```python
from build123d import *

# Parameters (mm, degrees)
SKETCH_1_W          = 8
SKETCH_1_H          = 5
EXTRUDE_1_DEPTH     = 5
SKETCH_2_W          = 1
SKETCH_2_H          = 2
EXTRUDE_2_DEPTH     = 5
EXTRUDE_3_DEPTH     = 1
SKETCH_7_W          = 8
SKETCH_7_H          = 1.5
EXTRUDE_4_DEPTH     = 1
CUT_EXTRUDE_2_DEPTH = 11.677078252
CUT_EXTRUDE_3_DEPTH = 10
CUT_EXTRUDE_4_DEPTH = 10
SKETCH_11_R         = 1.25
CUT_EXTRUDE_5_DEPTH = 1


with BuildPart() as part:
    # 草图1 → 凸台-拉伸1 (new body)
    with BuildSketch(Plane.XY):
        with Locations((0, 2.5)):
            Rectangle(SKETCH_1_W, SKETCH_1_H)
    extrude(amount=EXTRUDE_1_DEPTH)

    # 草图2 → 凸台-拉伸2 (add)
    with BuildSketch(Plane(origin=(0, 5, 0), x_dir=(1, 0, 0), z_dir=(0, 1, 0))):
        with Locations((-4.5, -2.5)):
            Rectangle(SKETCH_2_W, SKETCH_2_H)
        with Locations((4.5, -2.5)):
            Rectangle(SKETCH_2_W, SKETCH_2_H)
    extrude(amount=-EXTRUDE_2_DEPTH)

    # 草图6 → 凸台-拉伸3 (add, symmetric)
    with BuildSketch(Plane.XY.offset(2.5)):
        Polygon((4, 5), (4, 8), (-4, 5), align=None)
    extrude(amount=EXTRUDE_3_DEPTH, both=True)

    # 草图7 → 凸台-拉伸4 (add)
    with BuildSketch(Plane(origin=(0, 5, 0), x_dir=(1, 0, 0), z_dir=(0, 1, 0))):
        with Locations((0, -0.75)):
            Rectangle(SKETCH_7_W, SKETCH_7_H)
        with Locations((0, -4.25)):
            Rectangle(SKETCH_7_W, SKETCH_7_H)
    extrude(amount=EXTRUDE_4_DEPTH)

    # 草图8 → 切除-拉伸2 (cut, through all)
    with BuildSketch(Plane.XY.offset(5)):
        Polygon((-4, 5), (4, 8), (-4.143186706, 8), (-4.143186706, 5), align=None)
    extrude(amount=-CUT_EXTRUDE_2_DEPTH, mode=Mode.SUBTRACT)

    # 草图9 → 切除-拉伸3 (cut)
    with BuildSketch(Plane(origin=(0, 0, 1.5), x_dir=(-1, 0, 0), z_dir=(0, 0, -1))):
        Polygon((-4, 8), (-4, 5), (4, 5), align=None)
    extrude(amount=CUT_EXTRUDE_3_DEPTH, mode=Mode.SUBTRACT)

    # 草图10 → 切除-拉伸4 (cut)
    with BuildSketch(Plane.XY.offset(3.5)):
        Polygon((4, 8), (4, 5), (-4, 5), align=None)
    extrude(amount=CUT_EXTRUDE_4_DEPTH, mode=Mode.SUBTRACT)

    # 草图11 → 切除-拉伸5 (cut)
    with BuildSketch(Plane.XZ):
        with Locations(Location((0, 2.5, 0), (0, 0, 270))):
            Circle(SKETCH_11_R)
    extrude(amount=-CUT_EXTRUDE_5_DEPTH, mode=Mode.SUBTRACT)


solid = part.part
```
CAD build for the part. Positions are in the model's coordinates, mm. A direction names the side the tool comes from. Coordinates: 2 decimals unless noted, no trailing zeros. Write each loop counter-clockwise with the first axis right and the second up, starting at its lowest first coordinate (ties: lowest second). Pieces come first, ordered by that corner, then holes. Notation, with made-up numbers: (38, 84) -> (61, 84) arc R30 cw to (61, 114) -> close; hole circle Ø7 at (87.25, 86). An arc over 180 degrees is marked (long way). Return JSON: item names as keys, results as strings. Group by question number.
Q1. Pull direction Z, two halves, no side cores. Call faces 6 (the face through (-4.5, 2.5, 1.5)), 7 (the face through (0.38, 0.49, 1.31)), 8 (the face through (4, 2, 1)), 9 (the face through (0, 1, 3)): released by +Z, released by -Z, zero draft, split by the parting line, or undercut.
Q2. Cut at B-B, the plane z = 2.5. Give the cut face in (x, y).
Q3. Which spindle directions (+Z, -Z, +X, -X, +Y, -Y) get a long thin tool onto all of the face, cutting with end or side? Do faces 1 (the face through (4, 2, 4)), 2 (the face through (4.5, 5, 2.5)), 3 (the face through (0, 5, 4)), 4 (the face through (-4.5, 5, 2.5)), 5 (the face through (-4, 2, 4)). Say none if no direction does.
Q4. Flat gauge pins, fed straight in: pin 1 (0.6 mm diameter, centred on y = 7, z = 3, fed in from +X); pin 2 (0.8 mm diameter, centred on x = -4.5, y = 3.5, fed in from +Z); pin 3 (0.9 mm diameter, centred on x = -1.5, y = 7, fed in from -Z) (1 decimal); pin 4 (0.5 mm diameter, centred on x = -4.5, z = 2, fed in from +Y). Where does each tip first touch, or does it go through?
Q5. Drill centre lines: line 1 (X direction, y = 0.6, z = 2.5); line 2 (Z direction, x = 4.5, y = 2.25); line 3 (Y direction, x = -1, z = 4.3). Where is each one in solid material? Low to high.
Q6. Cut at A-A, the plane y = 2. Give the cut face in (x, z).
Q7. Cut at D-D, the plane x = -0.5. Give the cut face in (y, z).
Q8. Cut at C-C, the plane x = -3. Give the cut face in (y, z) (3 decimals).
Returned:
{
 "1": {"face 6": "released by -Z", "face 7": "undercut", "face 8": "zero draft", "face 9": "undercut"},
 "2": {"outline": "(-5, 0) -> (-1.25, 0) -> (-1.25, 1) -> (1.25, 1) -> (1.25, 0) -> (5, 0) -> (5, 5) -> (4, 5) -> (4, 8) -> (-4, 5) -> (-5, 5) -> close"},
 "3": {"face 1": "+Z, +X, +Y, -Y", "face 2": "+Z, -Z, +X, +Y", "face 3": "+Z, +X, -X, +Y", "face 4": "+Z, -Z, -X, +Y", "face 5": "+Z, -X, +Y, -Y"},
 "4": {"pin 1": "stops at x = 4", "pin 2": "stops at z = 3.5", "pin 3": "passes through", "pin 4": "stops at y = 5"},
 "5": {"line 1": "x = -5 to -1.25, 1.25 to 5", "line 2": "z = 1.5 to 3.5", "line 3": "y = 0 to 5"},
 "6": {"outline": "(-5, 1.5) -> (-4, 1.5) -> (-4, 0) -> (4, 0) -> (4, 1.5) -> (5, 1.5) -> (5, 3.5) -> (4, 3.5) -> (4, 5) -> (-4, 5) -> (-4, 3.5) -> (-5, 3.5) -> close"},
 "7": {"outline": "(0, 0) -> (5, 0) -> (5, 1.5) -> (6.31, 1.5) -> (6.31, 3.5) -> (5, 3.5) -> (5, 5) -> (0, 5) -> (0, 3.65) -> (1, 3.65) -> (1, 1.35) -> (0, 1.35) -> close"},
 "8": {"outline": "(0, 0) -> (5, 0) -> (5, 1.5) -> (5.375, 1.5) -> (5.375, 3.5) -> (5, 3.5) -> (5, 5) -> (0, 5) -> close"}
}
